Work out the finished part from the listing and answer in its coordinate system (mm). A direction names the side the tool comes from. Give positions to 0.01 mm unless a question says otherwise; leave off trailing zeros. Loops run counter-clockwise (first coordinate to the right, second up) from the corner with the lowest first, then second, coordinate; pieces in that order, holes last. Notation, with made-up numbers: (45.5, -2) - (62.5, -2) arc R5 ccw to (62.5, 4) - close; hole circle Ø8 at (25.5, 10.25). An arc over 180 degrees is marked (long way). One line per question, with ' | ' between items. Start each with the question number.
1. Section D-D (x = 7.5) is taken. Determine the outline of the cut face in (y, z).
2. Find the intervals of material crossed by line 1 (Y direction, x = 7.5, z = -16.5); line 2 (Y direction, x = 1.5, z = -8.75), in increasing order.
3. Section C-C (y = 39) is taken. Determine the outline of the cut face in (x, z).
4. Section B-B (z = -10) is taken. Determine the outline of the cut face in (x, y).
5. Which of the six approach directions +Z, -Z, +X, -X, +Y, -Y give full straight-line access (tool end or side, diameter ignored) to faces 1 (the face through (10, 45, -10)), 2 (the face through (12, 31.5, -12))?
6. Section A-A (x = 10) is taken. Determine the outline of the cut face in (y, z), plus the area to 4 significant figures.
from build123d import *

# Parameters (mm, degrees)
SKETCH1_W           = 20
SKETCH1_H           = 20
BOSS_EXTRUDE1_DEPTH = 30
SKETCH2_R           = 7.5
BOSS_EXTRUDE2_DEPTH = 1.5
SKETCH3_R           = 2
BOSS_EXTRUDE4_DEPTH = 13.5


with BuildPart() as part:
    # Sketch1 → Boss-Extrude1 (new body)
    with BuildSketch(Plane(origin=(0, 0, 0), x_dir=(1, 0, 0), z_dir=(0, 1, 0))):
        with Locations((10, 10)):
            Rectangle(SKETCH1_W, SKETCH1_H)
    extrude(amount=BOSS_EXTRUDE1_DEPTH)

    # Sketch2 → Boss-Extrude2 (add)
    with BuildSketch(Plane(origin=(0, 30, 0), x_dir=(1, 0, 0), z_dir=(0, 1, 0))):
        with Locations(Location((10, 10, 0), (0, 0, 90))):
            Circle(SKETCH2_R)
    extrude(amount=BOSS_EXTRUDE2_DEPTH)

    # Sketch3 → Boss-Extrude4 (add)
    with BuildSketch(Plane(origin=(0, 31.5, 0), x_dir=(1, 0, 0), z_dir=(0, 1, 0))):
        with Locations(Location((10, 10, 0), (0, 0, 270))):
            Circle(SKETCH3_R)
    extrude(amount=BOSS_EXTRUDE4_DEPTH)


solid = part.part
Conclusion:
1) outline: (0, -20) - (30, -20) - (30, -17.07) - (31.5, -17.07) - (31.5, -2.93) - (30, -2.93) - (30, 0) - (0, 0) - close
2) line 1: 0 to 31.5 | line 2: 0 to 30
3) outline: circle Ø4 at (10, -10)
4) outline: (0, 0) - (20, 0) - (20, 30) - (17.5, 30) - (17.5, 31.5) - (12, 31.5) - (12, 45) - (8, 45) - (8, 31.5) - (2.5, 31.5) - (2.5, 30) - (0, 30) - close
5) face 1: +Z, -Z, +X, -X, +Y | face 2: +Y
6) outline: (0, -20) - (30, -20) - (30, -17.5) - (31.5, -17.5) - (31.5, -12) - (45, -12) - (45, -8) - (31.5, -8) - (31.5, -2.5) - (30, -2.5) - (30, 0) - (0, 0) - close | area: 676.5 mm²
